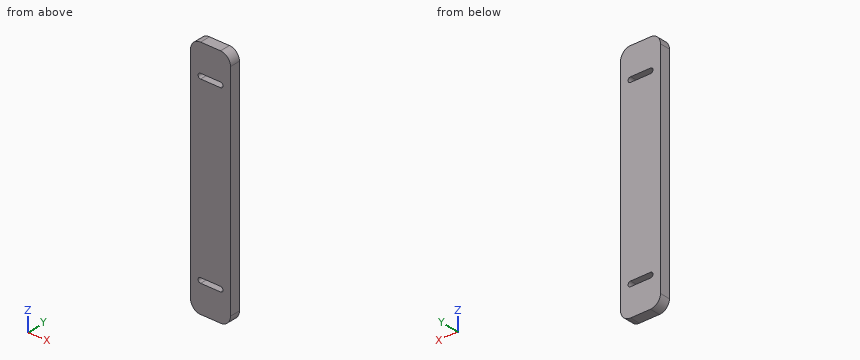
```python
from build123d import *

# Parameters (mm, degrees)
SKETCH1_W           = 25.4
SKETCH1_H           = 152.4
BOSS_EXTRUDE1_DEPTH = 6.604
CUT_EXTRUDE1_DEPTH  = 7.604
FILLET1_R           = 6.35


with BuildPart() as part:
    # Sketch1 → Boss-Extrude1 (new body)
    with BuildSketch(Plane(origin=(0, 0, 0), x_dir=(1, 0, 0), z_dir=(0, 1, 0))):
        Rectangle(SKETCH1_W, SKETCH1_H)
    extrude(amount=BOSS_EXTRUDE1_DEPTH)

    # Sketch2 → Cut-Extrude1 (cut, through all)
    with BuildSketch(Plane(origin=(0, 6.604, 0), x_dir=(1, 0, 0), z_dir=(0, 1, 0))):
        with BuildLine():
            Line((-6.35, 58.7375), (6.35, 58.7375))
            ThreePointArc((6.35, 58.7375), (7.9375, 57.15), (6.35, 55.5625))
            Line((6.35, 55.5625), (-6.35, 55.5625))
            ThreePointArc((-6.35, 55.5625), (-7.9375, 57.15), (-6.35, 58.7375))
        make_face()
        with BuildLine():
            Line((-6.35, -55.5625), (6.35, -55.5625))
            ThreePointArc((6.35, -55.5625), (7.9375, -57.15), (6.35, -58.7375))
            Line((6.35, -58.7375), (-6.35, -58.7375))
            ThreePointArc((-6.35, -58.7375), (-7.9375, -57.15), (-6.35, -55.5625))
        make_face()
    extrude(amount=-CUT_EXTRUDE1_DEPTH, mode=Mode.SUBTRACT)

    # Fillet1
    fillet1_edges = [part.edges().sort_by_distance(p)[0] for p in [
        (-12.7, 3.302, -76.2),
        (12.7, 3.302, -76.2),
        (12.7, 3.302, 76.2),
        (-12.7, 3.302, 76.2),
    ]]
    fillet(fillet1_edges, radius=FILLET1_R)


solid = part.part
```
The listing builds one solid part. Answer for the finished solid, in the listing's coordinates (mm). Coordinates: 2 decimals unless noted, no trailing zeros. Write each loop counter-clockwise with the first axis right and the second up, starting at its lowest first coordinate (ties: lowest second). Pieces come first, ordered by that corner, then holes.
Q1. Section C-C, the plane y = 1.25 is taken. Give the number of separate pieces and of enclosed holes in the cut face, then the cut area to 3 significant figures.
Returned:
separate pieces: 1
enclosed holes: 2
area: 3,740 mm2
Q2. Find the intervals of material crossed by line 1 along Z through (x, y) = (-6.5, 4.5); line 2 along Z through (x, y) = (7.5, 2.25) (3 decimals); line 3 along Z through (x, y) = (-8.5, 2.5), in increasing order.
Returned:
line 1: z = -76.2 to -58.73, -55.57 to 55.57, 58.73 to 76.2
line 2: z = -76.095 to -58.244, -56.056 to 56.056, 58.244 to 76.095
line 3: z = -75.82 to 75.82
Q3. Section A-A, the plane x = -3.25 is taken. Write down the section's boundary in (y, z), then the cut area to 3 significant figures.
Returned:
outline: (0, -76.2) - (6.6, -76.2) - (6.6, -58.74) - (0, -58.74) - close; (0, -55.56) - (6.6, -55.56) - (6.6, 55.56) - (0, 55.56) - close; (0, 58.74) - (6.6, 58.74) - (6.6, 76.2) - (0, 76.2) - close
area: 965 mm2
Q4. Section B-B, the plane z = 57.15 is taken. Write down the section's boundary in (x, y), then the cut area to 3 significant figures.
Returned:
outline: (-12.7, 0) - (-7.94, 0) - (-7.94, 6.6) - (-12.7, 6.6) - close; (7.94, 0) - (12.7, 0) - (12.7, 6.6) - (7.94, 6.6) - close
area: 62.9 mm2
